Geometry: final body of the model. Coordinates: model frame, mm. A direction names the side the tool comes from. Coordinates: 2 decimals unless noted, no trailing zeros. Loops run counter-clockwise (first coordinate to the right, second up) from the corner with the lowest first, then second, coordinate; pieces in that order, holes last. Notation, with made-up numbers: (-12, 32.25) -> (15, 32.25) arc R27 cw to (15, 65.25) -> close; hole circle Ø10 at (59.5, 53.25). An arc over 180 degrees is marked (long way). One line per item, written item: value. Start each with the question number.
from build123d import *

# Parameters (mm, degrees)
SKETCH1_R           = 4
BOSS_EXTRUDE1_DEPTH = 7.2
BOSS_EXTRUDE2_DEPTH = 4
SKETCH3_R           = 5
BOSS_EXTRUDE3_DEPTH = 3
CHAMFER1_SIZE       = 0.5
SKETCH4_R           = 10
BOSS_EXTRUDE4_DEPTH = 4
CHAMFER2_SIZE       = 0.2
SKETCH5_R           = 1.5
CUT_EXTRUDE1_DEPTH  = 24.048644212
SKETCH6_R           = 1.5
CUT_EXTRUDE2_DEPTH  = 4
SKETCH7_R           = 1.5
CUT_EXTRUDE3_DEPTH  = 4
CUT_EXTRUDE4_START  = -2
SKETCH7_3_R         = 1.5
CUT_EXTRUDE4_DEPTH  = 4
CUT_EXTRUDE5_DEPTH  = 5
CUT_EXTRUDE6_DEPTH  = 10


with BuildPart() as part:
    # Sketch1 → Boss-Extrude1 (new body)
    with BuildSketch(Plane(origin=(0, 0, 0), x_dir=(1, 0, 0), z_dir=(0, 1, 0))):
        with Locations(Location((0, 0, 0), (0, 0, 270))):
            Circle(SKETCH1_R)
    extrude(amount=BOSS_EXTRUDE1_DEPTH)

    # Sketch2 → Boss-Extrude2 (add)
    with BuildSketch(Plane(origin=(0, 7.2, 0), x_dir=(1, 0, 0), z_dir=(0, 1, 0))):
        Polygon((2, -3.464101615), (4, 0), (2, 3.464101615), (-2, 3.464101615), (-4, 0), (-2, -3.464101615), align=None)
    extrude(amount=BOSS_EXTRUDE2_DEPTH)

    # Sketch3 → Boss-Extrude3 (add)
    with BuildSketch(Plane.XZ):
        with Locations(Location((0, 0, 0), (0, 0, 270))):
            Circle(SKETCH3_R)
    extrude(amount=BOSS_EXTRUDE3_DEPTH)

    # Chamfer1
    chamfer1_edges = [part.edges().sort_by_distance(p)[0] for p in [
        (0, 0, 5),
    ]]
    chamfer(chamfer1_edges, length=CHAMFER1_SIZE)

    # Sketch4 → Boss-Extrude4 (add)
    with BuildSketch(Plane.XZ.offset(3)):
        with Locations(Location((0, 0, 0), (0, 0, 270))):
            Circle(SKETCH4_R)
    extrude(amount=BOSS_EXTRUDE4_DEPTH)

    # Chamfer2
    chamfer2_edges = [part.edges().sort_by_distance(p)[0] for p in [
        (0, -3, 10),
        (0, -7, 10),
    ]]
    chamfer(chamfer2_edges, length=CHAMFER2_SIZE)

    # Sketch5 → Cut-Extrude1 (cut, through all)
    with BuildSketch(Plane.XZ.offset(7)):
        with Locations(Location((0, 0, 0), (0, 0, 270))):
            Circle(SKETCH5_R)
    extrude(amount=-CUT_EXTRUDE1_DEPTH, mode=Mode.SUBTRACT)

    # Sketch6 → Cut-Extrude2 (cut)
    with BuildSketch(Plane.XZ.offset(7)):
        Polygon((2, -3.464101615), (4, 0), (2, 3.464101615), (-2, 3.464101615), (-4, 0), (-2, -3.464101615), align=None)
        with Locations(Location((0, 0, 0), (0, 0, 270))):
            Circle(SKETCH6_R, mode=Mode.SUBTRACT)
    extrude(amount=-CUT_EXTRUDE2_DEPTH, mode=Mode.SUBTRACT)

    # Sketch7 → Cut-Extrude3 (cut)
    with BuildSketch(Plane.XZ.offset(7)):
        with Locations(Location((-7, 0, 0), (0, 0, 270))):
            Circle(SKETCH7_R)
        with Locations(Location((0, -7, 0), (0, 0, 270))):
            Circle(SKETCH7_R)
        with Locations(Location((7, 0, 0), (0, 0, 270))):
            Circle(SKETCH7_R)
        with Locations(Location((0, 7, 0), (0, 0, 270))):
            Circle(SKETCH7_R)
    extrude(amount=-CUT_EXTRUDE3_DEPTH, mode=Mode.SUBTRACT)

    # Sketch7_3 → Cut-Extrude4 (cut)
    # profile 1 of 4: a face of its own
    with BuildSketch(Plane.XZ.offset(7).offset(CUT_EXTRUDE4_START)):
        Polygon((1.443375673, 4.5), (2.886751346, 7), (1.443375673, 9.5), (-1.443375673, 9.5), (-2.886751346, 7), (-1.443375673, 4.5), align=None)
        with Locations(Location((0, 7, 0), (0, 0, 270))):
            Circle(SKETCH7_3_R, mode=Mode.SUBTRACT)
    # profile 2 of 4: a face of its own
    with BuildSketch(Plane.XZ.offset(7).offset(CUT_EXTRUDE4_START)):
        Polygon((-4.5, 1.443375673), (-7, 2.886751346), (-9.5, 1.443375673), (-9.5, -1.443375673), (-7, -2.886751346), (-4.5, -1.443375673), align=None)
        with Locations(Location((-7, 0, 0), (0, 0, 270))):
            Circle(SKETCH7_3_R, mode=Mode.SUBTRACT)
    # profile 3 of 4: a face of its own
    with BuildSketch(Plane.XZ.offset(7).offset(CUT_EXTRUDE4_START)):
        Polygon((4.5, -1.443375673), (7, -2.886751346), (9.5, -1.443375673), (9.5, 1.443375673), (7, 2.886751346), (4.5, 1.443375673), align=None)
        with Locations(Location((7, 0, 0), (0, 0, 270))):
            Circle(SKETCH7_3_R, mode=Mode.SUBTRACT)
    # profile 4 of 4: a face of its own
    with BuildSketch(Plane.XZ.offset(7).offset(CUT_EXTRUDE4_START)):
        Polygon((-1.443375673, -4.5), (-2.886751346, -7), (-1.443375673, -9.5), (1.443375673, -9.5), (2.886751346, -7), (1.443375673, -4.5), align=None)
        with Locations(Location((0, -7, 0), (0, 0, 270))):
            Circle(SKETCH7_3_R, mode=Mode.SUBTRACT)
    extrude(amount=-CUT_EXTRUDE4_DEPTH, mode=Mode.SUBTRACT)

    # Sketch8 → Cut-Extrude5 (cut)
    with BuildSketch(Plane.XZ.offset(3)):
        Polygon((1.58771324, 2.75), (-1.58771324, 2.75), (-3.175426481, 0), (-1.58771324, -2.75), (1.58771324, -2.75), (3.175426481, 0), align=None)
    extrude(amount=-CUT_EXTRUDE5_DEPTH, mode=Mode.SUBTRACT)

    # Sketch9 → Cut-Extrude6 (cut)
    with BuildSketch(Plane.XZ.offset(7)):
        Polygon((8.485281374, 9.899494937), (5.656854249, 7.071067812), (7.071067812, 5.656854249), (9.899494937, 8.485281374), align=None)
    extrude(amount=-CUT_EXTRUDE6_DEPTH, mode=Mode.SUBTRACT)


solid = part.part
1. Pin query (flat end, axial travel): pin 1 Ø10 at (x, y) = (4.5, 7) entering from -Z; pin 2 Ø0.6 at (y, z) = (-4.5, -0.5) entering from +X; pin 3 Ø2.5 at (x, z) = (0, 0) entering from -Y; pin 4 Ø3 at (x, z) = (1, -7) entering from +Y. Return the tip coordinate at first contact, or that it passes through.
2. Section B-B on y = 3.75. Return the cut outline in (x, z).
3. Section A-A on y = 9.5. Return the cut outline in (x, z), plus the area to 3 significant figures.
4. Set-up query: faces 4 (the face through (6.354, -5.028, 6.374)), 5 (the face through (-3.014, -5.028, -1.708)), 6 (the face through (0, -3, 4.5)), 7 (the face through (0, -4, 9.5)), 8 (the face through (-3.014, 9.172, 1.708)). Return all of +Z, -Z, +X, -X, +Y, -Y with unobstructed straight access to the full face (end or side cutting, diameter ignored); none if empty.
5. Line query: L1, parallel to Y at x = 5, z = 4.25; L2, parallel to X at y = -5.55, z = 7; L3, parallel to X at y = -5.95, z = -7. Output: solid intervals per line, ascending. Write a range as [from, to].
6. Section C-C on x = 0.5. Count the separate pieces of the cut face and the enclosed holes in it, plus the area to 3 significant figures.
7. Draft query along Z for faces 1 (the face through (-3.905, 3.55, -0.867)), 2 (the face through (-2.155, -4.014, 8.268)), 3 (the face through (-4.2, -7, 0.1)). Return one class per face: released by +Z, released by -Z, zero draft, split by the parting line, or undercut.
Checks:
1. pin 1: z = -4
1. pin 2: x = 10
1. pin 3: through
1. pin 4: y = -5
2. outline: circle Ø8 at (0, 0); hole circle Ø3 at (0, 0)
3. outline: (-4, 0) -> (-2, -3.46) -> (2, -3.46) -> (4, 0) -> (2, 3.46) -> (-2, 3.46) -> close; hole circle Ø3 at (0, 0)
3. area: 34.5 mm²
4. face 4: +Y, -Y
4. face 5: -Y
4. face 6: none
4. face 7: +Y
4. face 8: +Z, -X, +Y
5. L1: [-7, -3]
5. L2: [-7.14, -1.5], [1.5, 5.73]
5. L3: [-7.14, -1.5], [1.5, 7.14]
6. separate pieces: 4
6. enclosed holes: 0
6. area: 79.8 mm²
7. face 1: split by the parting line
7. face 2: undercut
7. face 3: zero draft
